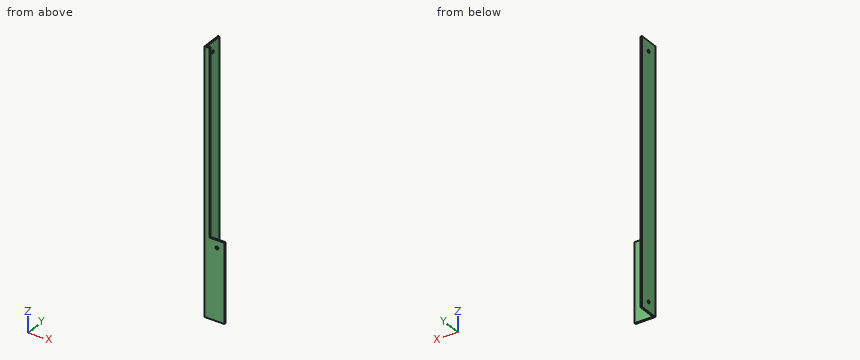
```python
from build123d import *

# Parameters (mm, degrees)
EXTRUSION1_DEPTH = 267
ESQUISSE2_R      = 1.5
ESQUISSE2_W      = 15
ESQUISSE2_H      = 187
EXTRUSION2_DEPTH = 269.38638192
ESQUISSE3_R      = 1.5
EXTRUSION3_DEPTH = 264


with BuildPart() as part:
    # Esquisse1 → Extrusion1 (new body)
    with BuildSketch(Plane.XY):
        Polygon((0, 0), (20, 0), (20, 1.5), (1.5, 1.5), (1.5, 20), (0, 20), align=None)
    extrude(amount=EXTRUSION1_DEPTH)

    # Esquisse2 → Extrusion2 (cut, through all)
    with BuildSketch(Plane(origin=(0, 1.5, 0), x_dir=(1, 0, 0), z_dir=(0, 1, 0))):
        with Locations(Location((12.5, -72.5, 0), (0, 0, 180))):
            Circle(ESQUISSE2_R)
        with Locations((12.5, -173.5)):
            Rectangle(ESQUISSE2_W, ESQUISSE2_H)
    extrude(amount=-EXTRUSION2_DEPTH, mode=Mode.SUBTRACT)

    # Esquisse3 → Extrusion3 (cut)
    with BuildSketch(Plane(origin=(1.5, 0, 0), x_dir=(0, 0, -1), z_dir=(1, 0, 0))):
        with Locations(Location((-257, 10, 0), (0, 0, 90))):
            Circle(ESQUISSE3_R)
        with Locations(Location((-10, 10, 0), (0, 0, 90))):
            Circle(ESQUISSE3_R)
    extrude(amount=-EXTRUSION3_DEPTH, mode=Mode.SUBTRACT)


solid = part.part
```
Check sheet for the modelled part. Datum: model origin and axes. Units: mm. Round coordinates to 2 decimals unless told otherwise and drop trailing zeros. Order: outer loops, then holes, each group sorted by start corner. A loop starts at its lowest first (then second) coordinate and runs counter-clockwise, first axis right, second up. Notation, with made-up numbers: (49.5, -38.5) -> (71.5, -38.5) arc R23 cw to (71.5, 0.5) -> close; hole circle Ø1 at (11, 84.25). An arc over 180 degrees is marked (long way). One line per item, written item: value. Start each with the question number.
Q1. Gauge pin test, flat ends, axial feed: pin 1 Ø9 at (y, z) = (15.5, 98.5) entering from +X; pin 2 Ø1.2 at (x, y) = (10.5, 1) entering from +Z; pin 3 Ø10 at (x, y) = (5, 17.5) entering from -Z; pin 4 Ø5 at (x, z) = (8, 56.5) entering from +Y. Record the tip position at first contact, or that the pin passes through.
Q2. Thickness scan on line 1 (Z direction, x = 0.4, y = 10); line 2 (Y direction, x = 1.05, z = 257); line 3 (Z direction, x = 12.5, y = 0.85). Record the ranges inside material, lowest first.
Q3. Cross-section at A-A (z = 109.5). Record the boundary of the cut face in (x, y), and give its area (4 significant figures).
Q4. Cross-section at B-B (y = 16). Record the boundary of the cut face in (x, z).
Completed:
1. pin 1: stops at x = 1.5
1. pin 2: stops at z = 80
1. pin 3: stops at z = 0
1. pin 4: stops at y = 1.5
2. line 1: z = 0 to 8.5, 11.5 to 255.5, 258.5 to 267
2. line 2: y = 0 to 8.5, 11.5 to 20
2. line 3: z = 0 to 71, 74 to 80
3. outline: (0, 0) -> (5, 0) -> (5, 1.5) -> (1.5, 1.5) -> (1.5, 20) -> (0, 20) -> close
3. area: 35.25 mm²
4. outline: (0, 0) -> (1.5, 0) -> (1.5, 267) -> (0, 267) -> close
